Geometry: final body of the model. Coordinates: model frame, mm. Round coordinates to 2 decimals unless told otherwise and drop trailing zeros. Order: outer loops, then holes, each group sorted by start corner. A loop starts at its lowest first (then second) coordinate and runs counter-clockwise, first axis right, second up. Notation, with made-up numbers: M 42.25,72.5 L 80.25,72.5 A20 cw 80.25,104.5 Z; hole C 13,-24.75 d4. An arc over 180 degrees is marked long. Return JSON: item names as keys, results as strings. Group by question number.
Q1. Cut plane C-C on z = -12.25. Output: boundary loops of the cut face in (x, y).
Q2. Cut plane A-A on z = 0. Output: boundary loops of the cut face in (x, y).
Q3. Contact query for flat-ended pins moving along their axis: pin 1 (0.6 mm diameter, centred on y = -1, z = -12, fed in from +X); pin 2 (0.6 mm diameter, centred on y = -0.5, z = -13, fed in from -X). Output: stop coordinate, or through.
Q4. Cut plane B-B on y = -0.9. Output: boundary loops of the cut face in (x, z), and give its area (3 significant figures).
Q5. Ray query, probe 1 along Z at (x, y) = (-4.5, -0.6); probe 2 along X at (y, z) = (-0.25, 0); probe 3 along X at (y, z) = (-1, -12.5). Return the intervals inside material, ascending.
Q6. Cut plane D-D on x = 4. Output: boundary loops of the cut face in (y, z), and give its area (3 significant figures).
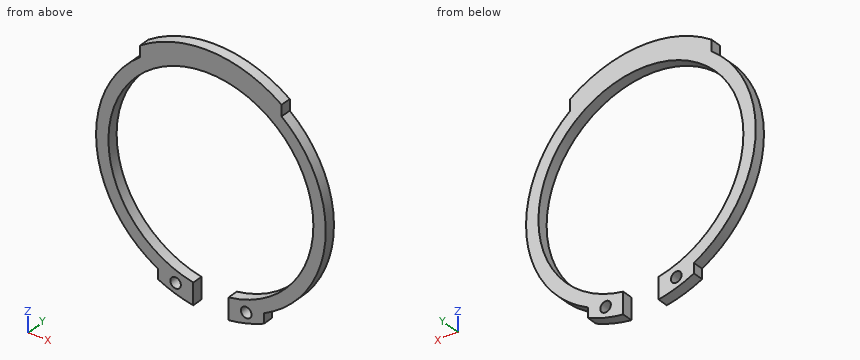
```python
from build123d import *

# Parameters (mm, degrees)
SKETCH_R  = 0.6
PAD_DEPTH = 1.2


with BuildPart() as part:
    # Sketch → Pad (new body)
    with BuildSketch(Plane.XZ):
        with BuildLine():
            ThreePointArc((2, -11.426285), (0, 11.6), (-2, -11.426285))
            Line((-2, -11.426285), (-2, -13.856406))
            ThreePointArc((-6, -12.649111), (-4.045292, -13.402821), (-2, -13.856406))
            Line((-6, -12.649111), (-6, -11.532563))
            ThreePointArc((-8, 10.246951), (-12.945532, -1.188781), (-6, -11.532563))
            Line((-8, 10.246951), (-8, 11.489125))
            ThreePointArc((8, 11.489125), (0, 14), (-8, 11.489125))
            Line((8, 10.246951), (8, 11.489125))
            ThreePointArc((6, -11.532563), (12.945532, -1.188781), (8, 10.246951))
            Line((6, -11.532563), (6, -12.649111))
            ThreePointArc((2, -13.856406), (4.045292, -13.402821), (6, -12.649111))
            Line((2, -11.426285), (2, -13.856406))
        make_face()
        with Locations((-4, -12.25)):
            Circle(SKETCH_R, mode=Mode.SUBTRACT)
        with Locations((4, -12.25)):
            Circle(SKETCH_R, mode=Mode.SUBTRACT)
    extrude(amount=PAD_DEPTH)


solid = part.part
```
Result sheet:
{
 "1": {"outline": "M -6,-1.2 L -4.6,-1.2 L -4.6,0 L -6,0 Z; M -3.4,-1.2 L -2,-1.2 L -2,0 L -3.4,0 Z; M 2,-1.2 L 3.4,-1.2 L 3.4,0 L 2,0 Z; M 4.6,-1.2 L 6,-1.2 L 6,0 L 4.6,0 Z"},
 "2": {"outline": "M -13,-1.2 L -11.6,-1.2 L -11.6,0 L -13,0 Z; M 11.6,-1.2 L 13,-1.2 L 13,0 L 11.6,0 Z"},
 "3": {"pin 1": "stops at x = 6", "pin 2": "stops at x = -5.89"},
 "4": {"outline": "M -8,10.25 A13 ccw -6,-11.53 L -6,-12.65 A14 ccw -2,-13.86 L -2,-11.43 A11.6 cw long 2,-11.43 L 2,-13.86 A14 ccw 6,-12.65 L 6,-11.53 A13 ccw 8,10.25 L 8,11.49 A14 ccw -8,11.49 Z; hole C -4,-12.25 d1.2; hole C 4,-12.25 d1.2", "area": "126 mm²"},
 "5": {"probe 1": "z = -13.26 to -12.58, -11.92 to -10.69, 10.69 to 13.26", "probe 2": "x = -13 to -11.6, 11.6 to 13", "probe 3": "x = -6 to -4.55, -3.45 to -2, 2 to 3.45, 4.55 to 6"},
 "6": {"outline": "M -1.2,-13.42 L 0,-13.42 L 0,-12.85 L -1.2,-12.85 Z; M -1.2,-11.65 L 0,-11.65 L 0,-10.89 L -1.2,-10.89 Z; M -1.2,10.89 L 0,10.89 L 0,13.42 L -1.2,13.42 Z", "area": "4.63 mm²"}
}
